The model under review builds one solid part; all positions refer to its coordinate system, in mm. A direction names the side the tool comes from. Round coordinates to 2 decimals unless told otherwise and drop trailing zeros. Order: outer loops, then holes, each group sorted by start corner. A loop starts at its lowest first (then second) coordinate and runs counter-clockwise, first axis right, second up.
Autodesk Inventor part; units mm, degrees
ref_plane "YZ Plane" through (0, 0, 0) normal (1, 0, 0) x (0, 1, 0)
ref_plane "XZ Plane" through (0, 0, 0) normal (0, 1, 0) x (-1, 0, 0)
ref_plane "XY Plane" through (0, 0, 0) normal (0, 0, 1) x (1, 0, 0)
sketch "Sketch1" plane through (0, 0, 0) normal (0, 1, 0) x (-1, 0, 0)
  line L0 (-16, 16.35) -> (16, 16.35)
  line L1 (16, 16.35) -> (16, -16.35)
  line L2 (16, -16.35) -> (-16, -16.35)
  line L3 (-16, -16.35) -> (-16, 16.35)
  line L4 (-16, 16.35) -> (16, -16.35) construction
  line L5 (16, 16.35) -> (-16, -16.35) construction
  point P0 (0, 0)
  dimension "d0" = 32
  dimension "d1" = 32.7
extrude "Extrusion1" add sketch "Sketch1" along normal blind 17
chamfer "Chamfer1" distance 2 angle 45 2 edges at (16, 8.5, 16.35) (16, 8.5, -16.35)
chamfer "Chamfer2" distance 2 angle 45 1 edges at (16, 8.5, -14.35)
sketch "Sketch3" plane through (16, 0, 14.35) normal (1, 0, 0) x (0, 0, -1)
  line L0 (-2, 17) -> (-2, 0)
  circle A0 centre (7.2, 8.5) radius 2.9
  point P0 (14.35, 0)
  point P1 (-2, 8.5)
  dimension "d10" = 9.2
  dimension "d11" = 5.8
extrude "Extrusion2" add sketch "Sketch3" along normal blind 5
sketch "Sketch4" plane through (-16, 0, 16.35) normal (0, 0, 1) x (1, 0, 0)
  line L0 (30, 17) -> (0, 17)
  line L1 (24.8, 17) -> (27, 17)
  line L2 (27, 17) -> (27, 0)
  line L3 (27, 0) -> (24.8, 0)
  line L4 (24.8, 0) -> (24.8, 17)
  line L5 (32, 0) -> (32, 17)
  point P0 (16, 0)
  point P1 (25.9, 0)
  dimension "d14" = 5
  dimension "d15" = 2.2
extrude "Extrusion3" add sketch "Sketch4" along normal blind 6.2
sketch "Sketch5" plane through (11, 0, 16.35) normal (1, 0, 0) x (0, 0, -1)
  line L0 (0, 17) -> (0, 0)
  line L1 (0, 17) -> (-6.2, 17)
  line L2 (-6.2, 0) -> (-6.2, 17)
  line L3 (0, 0) -> (-6.2, 0)
  line L4 (0, 17) -> (-6.2, 17) construction
  line L5 (-3.2, 17) -> (-3.2, 12.4994) construction
  line L6 (-3.2, 12.4994) -> (-3.2, 4.4994) construction
  line L7 (-3.2, 4.4994) -> (-3.1, 0) construction
  point P0 (16.35, 0)
  dimension "d18" = 3
  dimension "d19" = 8
hole "Hole1" at (11, 12.4994, 19.55) at (11, 4.4994, 19.55) direction (-1, 0, 0) diameter 4 depth 8 tip angle 118
sketch "Sketch6" plane through (-16, 0, -16.35) normal (0, 0, -1) x (-1, 0, 0)
  line L0 (-27, 17) -> (-24.8, 17)
  line L1 (-24.8, 17) -> (-24.8, 0)
  line L2 (-24.8, 0) -> (-27, 0)
  line L3 (-27, 0) -> (-27, 17)
  line L4 (-27, 17) -> (-24.8, 17)
  line L5 (-24.8, 17) -> (-24.8, 0)
  line L6 (-24.8, 0) -> (-27, 0)
  line L7 (-27, 0) -> (-27, 17)
  point P0 (-16, 0)
extrude "Extrusion4" add sketch "Sketch6" along normal blind 6.2
sketch "Sketch7" plane through (11, 0, -16.35) normal (1, 0, 0) x (0, 0, -1)
  circle A0 centre (-35.9, 12.4994) radius 2
  circle A1 centre (-35.9, 4.4994) radius 2
  line L0 (6.2, 17) -> (6.2, 0)
  point P0 (-16.35, 0)
  point P1 (3.2, 12.4994)
  point P2 (3.2, 4.4994)
  dimension "d29" = 3
hole "Hole2" at (11, 12.4994, -19.55) at (11, 4.4994, -19.55) direction (-1, 0, 0) diameter 4 depth 8 tip angle 118
chamfer "Chamfer3" distance 0.1 angle 45 1 edges at (21, 8.5, 10.05)
fillet "Fillet1" radius 0.5 4 edges at (-3.6, 17, 16.35) (-3.6, 17, -16.35) (-3.6, 0, 16.35) (-3.6, 0, -16.35)
hole "Hole3" at (21, 8.5, 7.15) direction (-1, 0, 0) diameter 2.459 depth 6 tip angle 118
properties part number "Corona-MG339MG"
(1) Insertion check: pin 1 (3.5 mm diameter, centred on y = 12.5, z = 19.55, fed in from +X); pin 2 (3.5 mm diameter, centred on x = 13, y = 7, fed in from -Z); pin 3 (5.5 mm diameter, centred on y = 12.5, z = -20, fed in from -X); pin 4 (8 mm diameter, centred on x = -1.5, y = 7, fed in from +Z). Each pin has a flat end and moves straight along its axis. Give the tip position at first contact, or say it passes through.
Data:
pin 1: passes through
pin 2: stops at z = -16.35
pin 3: stops at x = 8.8
pin 4: stops at z = 16.35
(2) To check wall thickness, follow probe 1 along Y at (x, z) = (9.5, -19.55); probe 2 along Y at (x, z) = (19.55, 7.15); probe 3 along X at (y, z) = (16.25, -9.5). State the ranges of each line that lie inside material, in increasing order.
Data:
probe 1: y = 0 to 2.5, 6.5 to 10.5, 14.5 to 17
probe 2: y = 5.6 to 7.27, 9.73 to 11.4
probe 3: x = -16 to 16
(3) Draft analysis for pull direction Z (two halves, no side actions). For faces 5 (the flat face through (10, 9, 22.55)), 6 (the cylindrical face through (18, 9.6, 6.6)), 7 (the cylindrical face through (18.42, 6.54, 9.29)), state which applies: pulls with the +Z half, pulls with the -Z half, needs draft (parallel to the pull), parting line crosses it, or undercut.
Data:
face 5: pulls with the +Z half
face 6: undercut
face 7: parting line crosses it
(4) Consider section C-C (y = 15.25). Write out the cut boundary in (x, z), and give its area (3 significant figures).
Data:
outline: (-16, -16.35) - (8.8, -16.35) - (8.8, -22.55) - (11, -22.55) - (11, -16.35) - (14, -16.35) - (14.59, -15.76) - (16, -12.35) - (16, 14.35) - (14, 16.35) - (11, 16.35) - (11, 22.55) - (8.8, 22.55) - (8.8, 16.35) - (-16, 16.35) - close
area: 1,070 mm2
(5) For faces 1 (the flat face through (11, 9, 19)), 2 (the flat face through (-3, 8, 16.35)), 3 (the flat face through (-4, 8, -16.35)), 4 (the flat face through (12, 8, -16.35)), list the 3-axis set-ups (+Z, -Z, +X, -X, +Y, -Y) from which the entire face can be reached by the end or side of a thin tool; tool diameter is ignored.
Data:
face 1: +Z, +X, +Y, -Y
face 2: +Z, -X, +Y, -Y
face 3: -Z, -X, +Y, -Y
face 4: -Z, +X, +Y, -Y
(6) Consider section A-A (z = -19.55). Write out the cut boundary in (x, y).
Data:
outline: (8.8, 0) - (11, 0) - (11, 2.5) - (8.8, 2.5) - close; (8.8, 6.5) - (11, 6.5) - (11, 10.5) - (8.8, 10.5) - close; (8.8, 14.5) - (11, 14.5) - (11, 17) - (8.8, 17) - close
(7) Consider section B-B (x = 2). Write out the cut boundary in (y, z).
Data:
outline: (0, -15.85) arc R0.5 ccw to (0.5, -16.35) - (16.5, -16.35) arc R0.5 ccw to (17, -15.85) - (17, 15.85) arc R0.5 ccw to (16.5, 16.35) - (0.5, 16.35) arc R0.5 ccw to (0, 15.85) - close
(8) Consider section D-D (z = -10). Write out the cut boundary in (x, y).
Data:
outline: (-16, 0) - (16, 0) - (16, 17) - (-16, 17) - close
